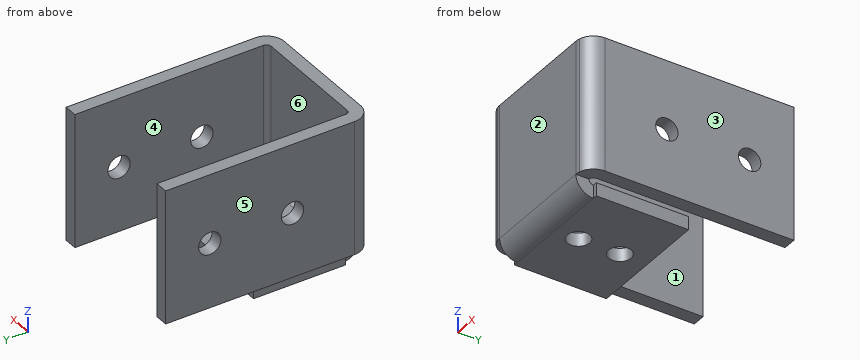
from build123d import *

# Parameters (mm, degrees)
SKETCH2_W                    = 45
SKETCH2_H                    = 50
BASE_FLANGE1_DEPTH           = 4.78
EDGE_FLANGE1_STRIP_W         = 22.32
EDGE_FLANGE1_STRIP_H         = 4.78
EDGE_FLANGE1_STRIP_CUT_DEPTH = 45
EDGE_FLANGE1_DEPTH           = 45
EDGE_FLANGE2_START           = -29.78
EDGE_FLANGE2_OUTLINE_W       = 1.6
EDGE_FLANGE2_OUTLINE_H       = 6.38
EDGE_FLANGE2_DEPTH           = 6.38
EDGE_FLANGE2_START_2         = -23.4
EDGE_FLANGE2_2_DEPTH         = 48.4
EDGE_FLANGE2_3_DEPTH         = 48.4
CUT_EXTRUDE1_REACH           = 95.614
SKETCH23_R                   = 4.05
SKETCH24_R                   = 4.05
CUT_EXTRUDE2_DEPTH           = 4.78


# Read off the part's stored shape, not the designer's step: Edge-Flange2
# Sheet-metal steps are written as plain solids
with BuildPart() as part:
    # Sketch2 → Base-Flange1 (new body)
    with BuildSketch(Plane(origin=(0, 0, 0), x_dir=(1, 0, 0), z_dir=(0, 1, 0))):
        Rectangle(SKETCH2_W, SKETCH2_H)
    extrude(amount=-BASE_FLANGE1_DEPTH)

    # Edge-Flange1 strip (across the edge) → Edge-Flange1 strip cut (cut)
    with BuildSketch(Plane(origin=(22.5, 0, -25), x_dir=(0, 0, 1), z_dir=(-1, 0, 0))):
        with Locations((-9.56, -2.39)):
            Rectangle(EDGE_FLANGE1_STRIP_W, EDGE_FLANGE1_STRIP_H)
    extrude(amount=EDGE_FLANGE1_STRIP_CUT_DEPTH, mode=Mode.SUBTRACT)

    # Edge-Flange1 section (across the edge) → Edge-Flange1 (add)
    with BuildSketch(Plane(origin=(22.5, 0, -25), x_dir=(0, 0, 1), z_dir=(-1, 0, 0))):
        with BuildLine():
            Line((-4.78, 1.6), (-4.78, 35))
            Line((-4.78, 35), (0, 35))
            Line((0, 35), (0, 1.6))
            ThreePointArc((0, 1.6), (0.46862915, 0.46862915), (1.6, 0))
            Line((1.6, 0), (1.6, -4.78))
            ThreePointArc((1.6, -4.78), (-2.911341264, -2.911341264), (-4.78, 1.6))
        make_face()
    extrude(amount=EDGE_FLANGE1_DEPTH)

    # Edge-Flange2 outline → Edge-Flange2 (cut)
    with BuildSketch(Plane.XY.offset(EDGE_FLANGE2_START)):
        with Locations((-21.7, -1.59)):
            Rectangle(EDGE_FLANGE2_OUTLINE_W, EDGE_FLANGE2_OUTLINE_H)
        with Locations((21.7, -1.59)):
            Rectangle(EDGE_FLANGE2_OUTLINE_W, EDGE_FLANGE2_OUTLINE_H)
    extrude(amount=EDGE_FLANGE2_DEPTH, mode=Mode.SUBTRACT)

    # Edge-Flange2 2 outline → Edge-Flange2 2 (cut)
    with BuildSketch(Plane.XY.offset(EDGE_FLANGE2_START_2)):
        with BuildLine():
            Line((-22.5, -4.78), (-20.9, -4.78))
            ThreePointArc((-20.9, -4.78), (-21.706468998, -4.728823568), (-22.5, -4.576115284))
            Line((-22.5, -4.576115284), (-22.5, -4.78))
        make_face()
        with BuildLine():
            ThreePointArc((22.5, -4.576115284), (21.706468998, -4.728823568), (20.9, -4.78))
            Line((20.9, -4.78), (22.5, -4.78))
            Line((22.5, -4.78), (22.5, -4.576115284))
        make_face()
    extrude(amount=EDGE_FLANGE2_2_DEPTH, mode=Mode.SUBTRACT)

    # Edge-Flange2 3 outline → Edge-Flange2 3 (add)
    with BuildSketch(Plane.XY.offset(EDGE_FLANGE2_START_2)):
        with BuildLine():
            Line((-22.5, -4.576115284), (-22.5, 0))
            Line((-22.5, 0), (-20.9, 0))
            ThreePointArc((-20.9, 0), (-22.03137085, 0.46862915), (-22.5, 1.6))
            Line((-22.5, 1.6), (-22.5, 70))
            Line((-22.5, 70), (-27.28, 70))
            Line((-27.28, 70), (-27.28, 1.6))
            ThreePointArc((-27.28, 1.6), (-25.945413759, -2.304894365), (-22.5, -4.576115284))
        make_face()
        with BuildLine():
            ThreePointArc((22.5, 1.6), (22.03137085, 0.46862915), (20.9, 0))
            Line((20.9, 0), (22.5, 0))
            Line((22.5, 0), (22.5, -4.576115284))
            ThreePointArc((22.5, -4.576115284), (25.945413759, -2.304894365), (27.28, 1.6))
            Line((27.28, 1.6), (27.28, 70))
            Line((27.28, 70), (22.5, 70))
            Line((22.5, 70), (22.5, 1.6))
        make_face()
    extrude(amount=EDGE_FLANGE2_3_DEPTH)

    # Cut-Extrude1: up to this face of the body (flat: up to its plane)
    cut_extrude1_end = Plane(part.part.faces().sort_by_distance((-27.28, 35.8, 0.8))[0])
    # Sketch23 → Cut-Extrude1 (cut, up to the picked face)
    with BuildSketch(Plane(origin=(27.28, 0, 0), x_dir=(0, 0, -1), z_dir=(1, 0, 0)), mode=Mode.PRIVATE) as cut_extrude1_sk1:
        with Locations(Location((0, 54, 0), (0, 0, 90))):
            Circle(SKETCH23_R)
    cut_extrude1_tool1 = split(extrude(cut_extrude1_sk1.sketch, amount=-CUT_EXTRUDE1_REACH, mode=Mode.PRIVATE), bisect_by=cut_extrude1_end, keep=Keep.BOTH, mode=Mode.PRIVATE)
    # Sketch23 → Cut-Extrude1 (cut, up to the picked face)
    with BuildSketch(Plane(origin=(27.28, 0, 0), x_dir=(0, 0, -1), z_dir=(1, 0, 0)), mode=Mode.PRIVATE) as cut_extrude1_sk2:
        with Locations(Location((0, 24, 0), (0, 0, 90))):
            Circle(SKETCH23_R)
    cut_extrude1_tool2 = split(extrude(cut_extrude1_sk2.sketch, amount=-CUT_EXTRUDE1_REACH, mode=Mode.PRIVATE), bisect_by=cut_extrude1_end, keep=Keep.BOTH, mode=Mode.PRIVATE)
    add(cut_extrude1_tool1.solids().sort_by(Axis((27.28, 54, 0), (-1, 0, 0)))[0], mode=Mode.SUBTRACT)
    add(cut_extrude1_tool2.solids().sort_by(Axis((27.28, 24, 0), (-1, 0, 0)))[0], mode=Mode.SUBTRACT)

    # Sketch24 → Cut-Extrude2 (cut)
    with BuildSketch(Plane(origin=(0, 0, -29.78), x_dir=(-1, 0, 0), z_dir=(0, 0, -1))):
        with Locations(Location((0, 25, 0), (0, 0, 90))):
            Circle(SKETCH24_R)
        with Locations(Location((0, 10, 0), (0, 0, 90))):
            Circle(SKETCH24_R)
    extrude(amount=-CUT_EXTRUDE2_DEPTH, mode=Mode.SUBTRACT)


solid = part.part
Build history of the part. All positions in model axes, mm. Face numbers are marked on the shaded views. A direction names the side the tool comes from. Give positions to 0.01 mm unless a question says otherwise; leave off trailing zeros. Write each loop counter-clockwise with the first axis right and the second up, starting at its lowest first coordinate (ties: lowest second). Pieces come first, ordered by that corner, then holes. Notation, with made-up numbers: (-29.75, 24) - (17.25, 24) arc R28 ccw to (17.25, 47) - close; hole circle Ø6 at (-14, -18). An arc over 180 degrees is marked (long way). Use one line per item in the form item = value. Start each with the question number.
1. 3-axis set-ups, long thin cutter, end or side, ignore diameter. For the marked faces 1 and 2: which of +Z, -Z, +X, -X, +Y, -Y reach the whole face in a straight line?
2. Band-saw the part on D-D on x = 16. Write the cut outline in (y, z).
3. Probe line 1 (X direction, y = 61.5, z = -14); line 2 (X direction, y = 25, z = -28); line 3 (Z direction, x = -24, y = 54). List the from-to ranges inside material, lowest first. Write a range as [from, to].
4. Band-saw the part on C-C on z = 0. Write the cut outline in (x, y), plus the area to 3 significant figures.
5. Drop flat-ended pins along their axis: pin 1 Ø5 at (y, z) = (24, 0) entering from +X; pin 2 Ø3 at (y, z) = (-3, -27) entering from -X; pin 3 Ø5 at (x, y) = (-25.5, 17) entering from -Z; pin 4 Ø5.5 at (y, z) = (22, -27.5) entering from +X. Give the stop position or say it passes through.
6. Two-plate mould, pull along X, no slides. Class the marked faces 3, 4, 5 and 6: released by +X, released by -X, zero draft, split by the parting line, or undercut.
7. Band-saw the part on B-B on y = 54. Write the cut outline in (x, z).
8. Band-saw the part on A-A on x = 0. Write the cut outline in (y, z), plus the area to 3 significant figures.
Conclusion:
q1.face_1 = +Z, +Y
q1.face_2 = +Z, -Z, +X, -X, -Y
q2.outline = (-4.78, -23.4) arc R6.38 ccw to (1.6, -29.78) - (35, -29.78) - (35, -25) - (1.6, -25) arc R1.6 cw to (0, -23.4) - (0, 25) - (-4.78, 25) - close
q3.line_1 = [-27.28, -22.5], [22.5, 27.28]
q3.line_2 = [-22.5, -4.05], [4.05, 22.5]
q3.line_3 = [-23.4, -4.05], [4.05, 25]
q4.outline = (-27.28, 1.6) arc R6.38 ccw to (-20.9, -4.78) - (20.9, -4.78) arc R6.38 ccw to (27.28, 1.6) - (27.28, 19.95) - (22.5, 19.95) - (22.5, 1.6) arc R1.6 cw to (20.9, 0) - (-20.9, 0) arc R1.6 cw to (-22.5, 1.6) - (-22.5, 19.95) - (-27.28, 19.95) - close; (-27.28, 28.05) - (-22.5, 28.05) - (-22.5, 49.95) - (-27.28, 49.95) - close; (-27.28, 58.05) - (-22.5, 58.05) - (-22.5, 70) - (-27.28, 70) - close; (22.5, 28.05) - (27.28, 28.05) - (27.28, 49.95) - (22.5, 49.95) - close; (22.5, 58.05) - (27.28, 58.05) - (27.28, 70) - (22.5, 70) - close
q4.area = 759 mm²
q5.pin_1 = through
q5.pin_2 = -20.9
q5.pin_3 = -23.4
q5.pin_4 = 22.5
q6.face_3 = released by +X
q6.face_4 = undercut
q6.face_5 = released by -X
q6.face_6 = undercut
q7.outline = (-27.28, -23.4) - (-22.5, -23.4) - (-22.5, -4.05) - (-27.28, -4.05) - close; (-27.28, 4.05) - (-22.5, 4.05) - (-22.5, 25) - (-27.28, 25) - close; (22.5, -23.4) - (27.28, -23.4) - (27.28, -4.05) - (22.5, -4.05) - close; (22.5, 4.05) - (27.28, 4.05) - (27.28, 25) - (22.5, 25) - close
q8.outline = (-4.78, -23.4) arc R6.38 ccw to (1.6, -29.78) - (5.95, -29.78) - (5.95, -25) - (1.6, -25) arc R1.6 cw to (0, -23.4) - (0, 25) - (-4.78, 25) - close; (14.05, -29.78) - (20.95, -29.78) - (20.95, -25) - (14.05, -25) - close; (29.05, -29.78) - (35, -29.78) - (35, -25) - (29.05, -25) - close
q8.area = 344 mm²
